Can you work these out from the model? Positions are in its coordinate system, mm. A direction names the side the tool comes from. Give positions to 0.01 mm unless a question says otherwise; leave off trailing zeros. Order: outer loops, then holes, each group sorted by start corner. A loop starts at its lowest first (then second) coordinate and runs counter-clockwise, first axis right, second up. Notation, with made-up numbers: (3, -27.5) -> (59, -27.5) arc R33 ccw to (59, 9.5) -> close; hole circle Ø3 at (27.5, -19). An arc over 180 degrees is marked (long way). Answer as a JSON object with one key per item and string values.
```python
from build123d import *

# Parameters (mm, degrees)
SKETCH_1_R               = 18
SKETCH_1_R_2             = 1
EXTRUDE_1_DEPTH          = 4
EXTRUDE_2_DEPTH          = 20
PATTERN_CIRCULAR_1_COUNT = 4
SKETCH_3_R               = 1.575
EXTRUDE_3_DEPTH          = 1.5
PATTERN_CIRCULAR_2_COUNT = 4
SKETCH_4_R               = 6.25
CUT_EXTRUDE_1_DEPTH      = 2
CHAMFER_1_SIZE           = 0.5


with BuildPart() as part:
    # ｽｹｯﾁ1 → ﾎﾞｽ - 押し出し1 (new body)
    with BuildSketch(Plane.XY):
        Circle(SKETCH_1_R)
        with Locations((0, 3)):
            Circle(SKETCH_1_R_2, mode=Mode.SUBTRACT)
        with Locations((3, 0)):
            Circle(SKETCH_1_R_2, mode=Mode.SUBTRACT)
        with Locations((0, -3)):
            Circle(SKETCH_1_R_2, mode=Mode.SUBTRACT)
        with Locations((-3, 0)):
            Circle(SKETCH_1_R_2, mode=Mode.SUBTRACT)
    extrude(amount=EXTRUDE_1_DEPTH)

    # ｽｹｯﾁ2 → ﾎﾞｽ - 押し出し2 (add)
    with BuildSketch(Plane.XY.offset(4)):
        with BuildLine():
            Line((16.313540167, -7.607128711), (11.782001231, -5.494037403))
            ThreePointArc((11.782001231, -5.494037403), (9.192388155, -9.192388155), (5.494037403, -11.782001231))
            Line((5.494037403, -11.782001231), (7.607128711, -16.313540167))
            ThreePointArc((7.607128711, -16.313540167), (12.727922061, -12.727922061), (16.313540167, -7.607128711))
        make_face()
    extrude_2 = extrude(amount=EXTRUDE_2_DEPTH)

    # 円形ﾊﾟﾀｰﾝ1: ﾎﾞｽ - 押し出し2 ×4 about axis
    pattern_circular_1_axis = Axis((0, 0, 24), (0, 0, -1))
    for i in range(1, PATTERN_CIRCULAR_1_COUNT):
        add(extrude_2.rotate(pattern_circular_1_axis, i * 360 / PATTERN_CIRCULAR_1_COUNT))

    # ｽｹｯﾁ3 → ﾎﾞｽ - 押し出し3 (add)
    with BuildSketch(Plane.XY.offset(24)):
        with Locations((8.485281374, 12.727922061)):
            Circle(SKETCH_3_R)
        with Locations((12.727922061, 8.485281374)):
            Circle(SKETCH_3_R)
    extrude_3 = extrude(amount=EXTRUDE_3_DEPTH)

    # 円形ﾊﾟﾀｰﾝ2: ﾎﾞｽ - 押し出し3 ×4 about axis
    pattern_circular_2_axis = Axis((0, 0, 0), (0, 0, 1))
    for i in range(1, PATTERN_CIRCULAR_2_COUNT):
        add(extrude_3.rotate(pattern_circular_2_axis, i * 360 / PATTERN_CIRCULAR_2_COUNT))

    # ｽｹｯﾁ4 → ｶｯﾄ - 押し出し1 (cut)
    with BuildSketch(Plane(origin=(0, 0, 0), x_dir=(-1, 0, 0), z_dir=(0, 0, -1))):
        Circle(SKETCH_4_R)
    extrude(amount=-CUT_EXTRUDE_1_DEPTH, mode=Mode.SUBTRACT)

    # 面取り1
    chamfer_1_edges = [part.edges().sort_by_distance(p)[0] for p in [
        (6.910281374, 12.727922061, 25.5),
        (11.152922061, 8.485281374, 25.5),
        (12.727922061, -6.910281374, 25.5),
        (8.485281374, -11.152922061, 25.5),
        (-6.910281374, -12.727922061, 25.5),
        (-11.152922061, -8.485281374, 25.5),
        (-12.727922061, 6.910281374, 25.5),
        (-8.485281374, 11.152922061, 25.5),
    ]]
    chamfer(chamfer_1_edges, length=CHAMFER_1_SIZE)


solid = part.part
```
1. If we section it at C-C on x = -3: Please give me the cut outline in (y, z), then the cut area to 3 significant figures.
Worked answers:
{"outline": "(-17.75, 0) -> (-5.48, 0) -> (-5.48, 2) -> (-1, 2) -> (-1, 4) -> (-17.75, 4) -> close; (1, 2) -> (5.48, 2) -> (5.48, 0) -> (17.75, 0) -> (17.75, 4) -> (1, 4) -> close", "area": "116 mm²"}
2. Will these pins go through, and if not, where does the flat tip stop? pin 1 Ø14 at (x, y) = (2.5, 0.5) entering from -Z; pin 2 Ø5 at (x, z) = (-6, 4) entering from +Y; pin 3 Ø2 at (y, z) = (9, 14) entering from +X; pin 4 Ø4 at (x, z) = (14, 4.5) entering from +Y.
Worked answers:
{"pin 1": "z = 0", "pin 2": "y = 17.66", "pin 3": "x = 16.12", "pin 4": "y = 13.42"}
3. For faces 4 (the face through (-5.96, 1.88, 0.99)), 5 (the face through (14.079, -6.565, 13.86)), 6 (the face through (-14.016, -6.536, 13.86)), 7 (the face through (6.536, -14.016, 13.86)), 8 (the face through (12.8, -6.91, 24.49)), which set-ups out of +Z, -Z, +X, -X, +Y, -Y let a thin tool reach every point of the face, with its end or its side?
Worked answers:
{"face 4": "-Z", "face 5": "+Z, +X", "face 6": "+Z, -X", "face 7": "+Z, -Y", "face 8": "+Z"}
4. If we section it at A-A on z = 7.25: Please give me the cut outline in (x, y).
Worked answers:
{"outline": "(-16.31, -7.61) arc R18 ccw to (-7.61, -16.31) -> (-5.49, -11.78) arc R13 cw to (-11.78, -5.49) -> close; (-16.31, 7.61) -> (-11.78, 5.49) arc R13 cw to (-5.49, 11.78) -> (-7.61, 16.31) arc R18 ccw to start; (5.49, -11.78) -> (7.61, -16.31) arc R18 ccw to (16.31, -7.61) -> (11.78, -5.49) arc R13 cw to start; (5.49, 11.78) arc R13 cw to (11.78, 5.49) -> (16.31, 7.61) arc R18 ccw to (7.61, 16.31) -> close"}
5. If we mould it in two halves opening along Y, with no side actions, what happens to faces 1 (the face through (-11, -11, 24)), 2 (the face through (-6.565, -14.079, 13.86)), 3 (the face through (-13, -9, 25.5))? For each: +Y half, -Y half, draft (parallel to the pull), parting line (faces both ways), or undercut.
Worked answers:
{"face 1": "undercut", "face 2": "-Y half", "face 3": "draft"}
6. If we section it at B-B on y = 0: Please give me the cut outline in (x, z), then the cut area to 3 significant figures.
Worked answers:
{"outline": "(-18, 0) -> (-6.25, 0) -> (-6.25, 2) -> (-4, 2) -> (-4, 4) -> (-18, 4) -> close; (-2, 2) -> (2, 2) -> (2, 4) -> (-2, 4) -> close; (4, 2) -> (6.25, 2) -> (6.25, 0) -> (18, 0) -> (18, 4) -> (4, 4) -> close", "area": "111 mm²"}
7. If we section it at D-D on x = 5: Please give me the cut outline in (y, z), then the cut area to 3 significant figures.
Worked answers:
{"outline": "(-17.29, 0) -> (-3.75, 0) -> (-3.75, 2) -> (3.75, 2) -> (3.75, 0) -> (17.29, 0) -> (17.29, 4) -> (-17.29, 4) -> close", "area": "123 mm²"}
8. Please list where these lines run through material, in increasing order: L1, parallel to Y at x = 0, z = 2.4; L2, parallel to Y at x = 0, z = 1; L3, parallel to Z at x = 16, y = 1.
Worked answers:
{"L1": "-18 to -4, -2 to 2, 4 to 18", "L2": "-18 to -6.25, 6.25 to 18", "L3": "0 to 4"}
